Study the drawing (mm; zero at the part's minimum x, y, z) and answer. A direction names the side the tool comes from. Round coordinates to 2 decimals unless told otherwise and drop trailing zeros. Loops run counter-clockwise (first coordinate to the right, second up) from the corner with the lowest first, then second, coordinate; pieces in that order, holes last. Notation, with made-up numbers: (-37, -14.5) -> (-7, -14.5) arc R15 cw to (-7, -0.5) -> close; hole circle Ø8 at (66.25, 24). An arc over 180 degrees is marked (long way). Write each question's results on one line, items separated by ' | '. Start each with the question number.
(1) The part is cut by section B-B (y = 52.5). Determine the outline of the cut face in (x, z).
(2) Determine the mould class of the marked faces 1, 2, 3 and 4 for opening direction X: released by +X, released by -X, zero draft, split by the parting line, or undercut.
(3) The part is cut by section D-D (x = 392). Determine the outline of the cut face in (y, z).
(4) The part is cut by section A-A (x = 203). Determine the outline of the cut face in (y, z).
(5) The part is cut by section C-C (z = 153). Determine the outline of the cut face in (x, y), plus the area to 4 significant figures.
(6) Straight lines are drawn through the part: probe 1 along X at (y, z) = (75, 123); probe 2 along X at (y, z) = (83.5, 15); probe 3 along Z at (x, y) = (441, 74.75). For each, find the intervals that lie inside material, in ascending order.
(7) Flat-ended cylindrical pins translate along their axes: pin 1 (9.5 mm diameter, centred on x = 109, z = 191, fed in from +Y); pin 2 (7 mm diameter, centred on x = 109, z = 123, fed in from -Y); pin 3 (3 mm diameter, centred on x = 169.5, z = 15.5, fed in from +Y). Find the tip coordinate at first contact, or state that the pin passes through.
(8) For the marked faces 5 and 6, determine the directions among +Z, -Z, +X, -X, +Y, -Y from which every point of the face is accessible in a straight line to the end or side of a thin tool.
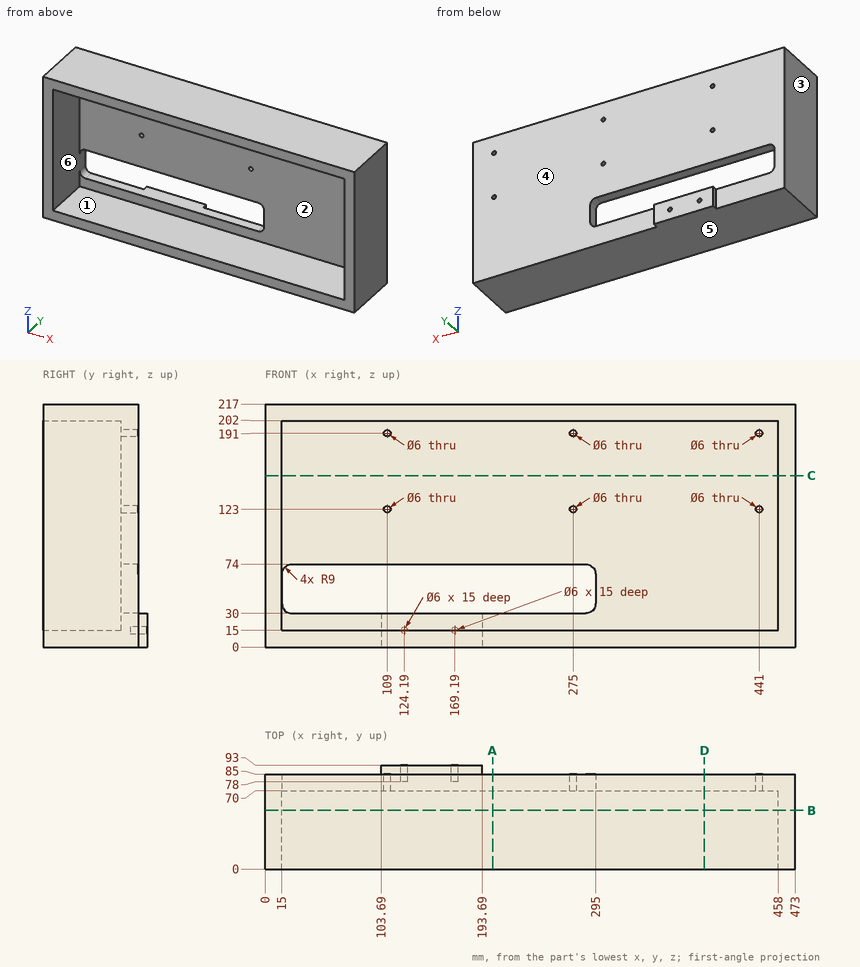
Checked values:
1) outline: (0, 0) -> (473, 0) -> (473, 217) -> (0, 217) -> close; hole (15, 15) -> (458, 15) -> (458, 202) -> (15, 202) -> close
2) face 1: undercut | face 2: undercut | face 3: released by -X | face 4: zero draft
3) outline: (0, 0) -> (85, 0) -> (85, 217) -> (0, 217) -> (0, 202) -> (70, 202) -> (70, 15) -> (0, 15) -> close
4) outline: (0, 0) -> (85, 0) -> (85, 30) -> (70, 30) -> (70, 15) -> (0, 15) -> close; (0, 202) -> (70, 202) -> (70, 74) -> (85, 74) -> (85, 217) -> (0, 217) -> close
5) outline: (0, 0) -> (15, 0) -> (15, 70) -> (458, 70) -> (458, 0) -> (473, 0) -> (473, 85) -> (0, 85) -> close | area: 9,195 mm2
6) probe 1: x = 0 to 106, 112 to 272, 278 to 438, 444 to 473 | probe 2: x = 0 to 121.19, 127.19 to 166.19, 172.19 to 473 | probe 3: z = 0 to 120, 126 to 188, 194 to 217
7) pin 1: stops at y = 85 | pin 2: stops at y = 70 | pin 3: stops at y = 78
8) face 5: -Z, +X, -X, +Y, -Y | face 6: -Y
